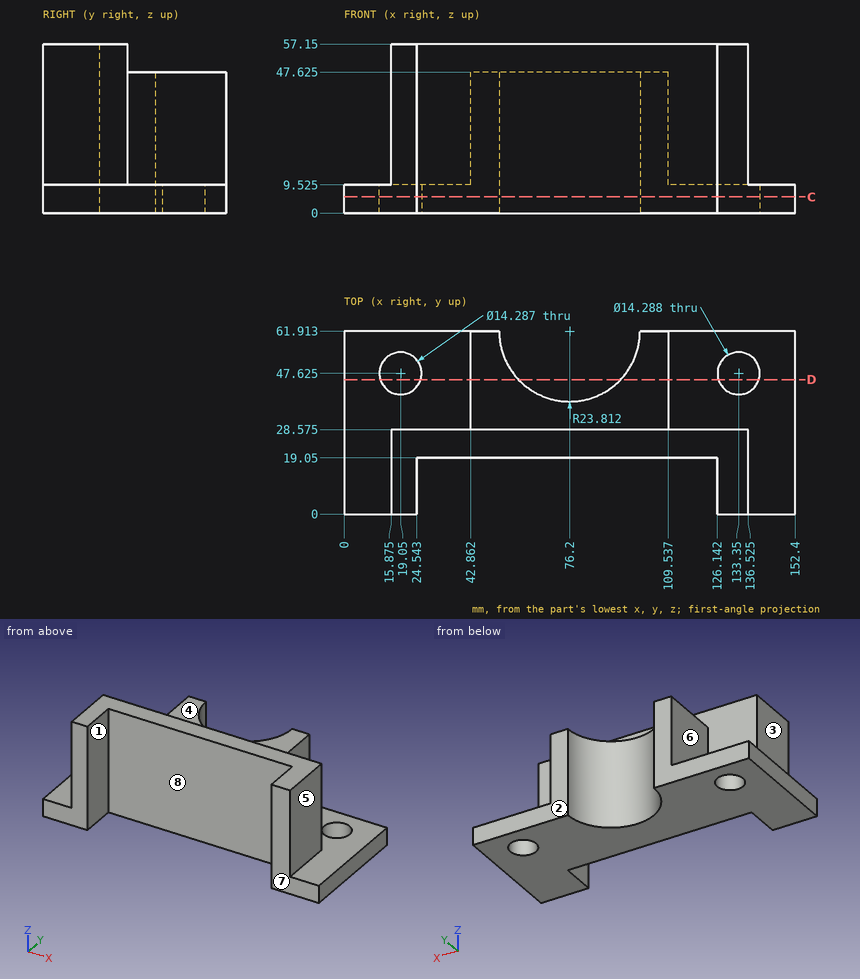
The drawing under review shows one solid part. Ordinate dimensions are in mm from its lowest x, y, z. A direction names the side the tool comes from. Round coordinates to 2 decimals unless told otherwise and drop trailing zeros. Loops run counter-clockwise (first coordinate to the right, second up) from the corner with the lowest first, then second, coordinate; pieces in that order, holes last. Notation, with made-up numbers: (61, -29.5) -> (80, -29.5) arc R33 ccw to (80, 3.5) -> close; hole circle Ø11 at (21, -3.75). An arc over 180 degrees is marked (long way). One line per question, with ' | ' between items. Start each with the question number.
Item 1: Machinability: for the marked faces 1, 2, 3 and 4, which of the approach directions +Z, -Z, +X, -X, +Y, -Y give a long, thin tool a straight path to every point of the face, cutting with its end or side? Answer none if there is none.
Item 2: Wall thickness on line 1 along Y through (x, z) = (19, 2); line 2 along X through (y, z) = (11, 30.5) (1 decimal); line 3 along X through (y, z) = (36, 15.5): over which ranges is each line inside the solid? List them lowest first. Write a range as [from, to].
Item 3: Add section C-C, the plane z = 5.5. Count the separate pieces of the cut face and the enclosed holes in it, then the cut area to 3 significant figures.
Item 4: Add section D-D, the plane y = 45.5. Write out the cut boundary in (x, z) (1 decimal), then the cut area to 3 significant figures.
Item 5: For pin 1 (8 mm diameter, centred on x = 77, z = 21.5, fed in from +Y); pin 2 (10 mm diameter, centred on x = 82, z = 28, fed in from -Y); pin 3 (23 mm diameter, centred on x = 133.35, y = 47.625, fed in from -Z); pin 4 (12 mm diameter, centred on y = 11, z = 43.5, fed in from +X) (1 decimal), all flat-tipped, find the tip position at first contact; note any pin that passes through.
Item 6: Draft analysis for pull direction X (two halves, no side actions). For the marked faces 5, 6, 7 and 8, state which applies: +X half, -X half, draft (parallel to the pull), parting line (faces both ways), or undercut.
Return value:
1) face 1: +Z, -Z, -Y | face 2: +Z, -Z, +X, -X, +Y | face 3: +Z, -X, +Y, -Y | face 4: +Z, +X, -X, +Y
2) line 1: y = [0, 40.48], [54.77, 61.91] | line 2: x = [15.9, 24.5], [126.1, 136.5] | line 3: x = [42.86, 109.54]
3) separate pieces: 1 | enclosed holes: 2 | area: 6,290 mm2
4) outline: (0, 0) -> (12.2, 0) -> (12.2, 9.5) -> (0, 9.5) -> close; (25.9, 0) -> (58.9, 0) -> (58.9, 47.6) -> (42.9, 47.6) -> (42.9, 9.5) -> (25.9, 9.5) -> close; (93.5, 0) -> (126.5, 0) -> (126.5, 9.5) -> (109.5, 9.5) -> (109.5, 47.6) -> (93.5, 47.6) -> close; (140.2, 0) -> (152.4, 0) -> (152.4, 9.5) -> (140.2, 9.5) -> close | area: 2,090 mm2
5) pin 1: stops at y = 38.59 | pin 2: stops at y = 19.05 | pin 3: stops at z = 0 | pin 4: stops at x = 136.5
6) face 5: +X half | face 6: -X half | face 7: draft | face 8: undercut
